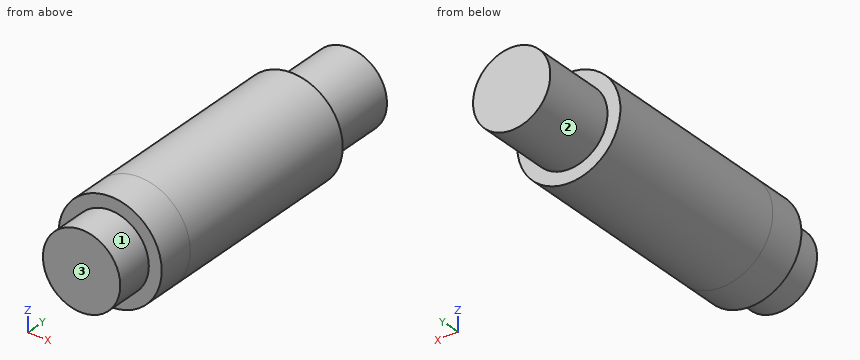
from build123d import *

# Parameters (mm, degrees)
SKETCH1_R           = 20
BOSS_EXTRUDE1_DEPTH = 40
SKETCH2_R           = 15
BOSS_EXTRUDE2_DEPTH = 30
SKETCH3_R           = 15
BOSS_EXTRUDE3_DEPTH = 30
SKETCH4_R           = 20
BOSS_EXTRUDE4_DEPTH = 15


with BuildPart() as part:
    # Sketch1 → Boss-Extrude1 (new body, symmetric)
    with BuildSketch(Plane(origin=(0, 0, 0), x_dir=(1, 0, 0), z_dir=(0, 1, 0))):
        Circle(SKETCH1_R)
    extrude(amount=BOSS_EXTRUDE1_DEPTH, both=True)

    # Sketch2 → Boss-Extrude2 (add)
    with BuildSketch(Plane(origin=(0, 40, 0), x_dir=(1, 0, 0), z_dir=(0, 1, 0))):
        Circle(SKETCH2_R)
    extrude(amount=BOSS_EXTRUDE2_DEPTH)

    # Sketch3 → Boss-Extrude3 (add)
    with BuildSketch(Plane.XZ.offset(40)):
        Circle(SKETCH3_R)
    extrude(amount=BOSS_EXTRUDE3_DEPTH)

    # Sketch4 → Boss-Extrude4 (add)
    with BuildSketch(Plane.XZ.offset(40)):
        Circle(SKETCH4_R)
    extrude(amount=BOSS_EXTRUDE4_DEPTH)


solid = part.part
Build history of the part. All positions in model axes, mm. Face numbers are marked on the shaded views. A direction names the side the tool comes from. Give positions to 0.01 mm unless a question says otherwise; leave off trailing zeros. Order: outer loops, then holes, each group sorted by start corner. A loop starts at its lowest first (then second) coordinate and runs counter-clockwise, first axis right, second up. Notation, with made-up numbers: M 10,38.25 L 67,38.25 A17 ccw 67,64.25 Z; hole C 55.25,39 d9. An arc over 180 degrees is marked long. Put each result on its own line as item: value.
Item 1: Slice it at A-A, the plane x = 0. Write the cut outline in (y, z).
From the geometry:
outline: M -70,-15 L -55,-15 L -55,-20 L 40,-20 L 40,-15 L 70,-15 L 70,15 L 40,15 L 40,20 L -55,20 L -55,15 L -70,15 Z
Item 2: 3-axis set-ups, long thin cutter, end or side, ignore diameter. For the marked faces 1, 2 and 3: which of +Z, -Z, +X, -X, +Y, -Y reach the whole face in a straight line?
From the geometry:
face 1: -Y
face 2: +Y
face 3: +Z, -Z, +X, -X, -Y
Item 3: Slice it at C-C, the plane y = 4. Write the cut outline in (x, z), plus the area to 3 significant figures.
From the geometry:
outline: C 0,0 d40
area: 1,260 mm2
Item 4: Probe line 1 (Y direction, x = -17, z = 5); line 2 (X direction, y = 30, z = 1); line 3 (Z direction, x = -13, y = 12.5). List the from-to ranges inside material, lowest first. Write a range as [from, to].
From the geometry:
line 1: y = [-55, 40]
line 2: x = [-19.97, 19.97]
line 3: z = [-15.2, 15.2]
Item 5: Flat gauge pins, fed straight in: pin 1 Ø1.5 at (y, z) = (-15.5, 9) entering from -X; pin 2 Ø1.5 at (y, z) = (6.5, -2) entering from -X; pin 3 Ø8 at (y, z) = (28, -11) entering from -X (3 decimals); pin 4 Ø3 at (x, z) = (-12, -9.5) entering from +Y. Where does each tip first touch, or does it go through?
From the geometry:
pin 1: stops at x = -18.22
pin 2: stops at x = -19.96
pin 3: stops at x = -18.735
pin 4: stops at y = 70
Item 6: Slice it at B-B, the plane z = 0. Write the cut outline in (x, y), plus the area to 3 significant figures.
From the geometry:
outline: M -20,-55 L -15,-55 L -15,-70 L 15,-70 L 15,-55 L 20,-55 L 20,40 L 15,40 L 15,70 L -15,70 L -15,40 L -20,40 Z
area: 5,150 mm2
